The model under review builds one solid part; all positions refer to its coordinate system, in mm. Give positions to 0.01 mm unless a question says otherwise; leave off trailing zeros. Order: outer loops, then holes, each group sorted by start corner. A loop starts at its lowest first (then second) coordinate and runs counter-clockwise, first axis right, second up.
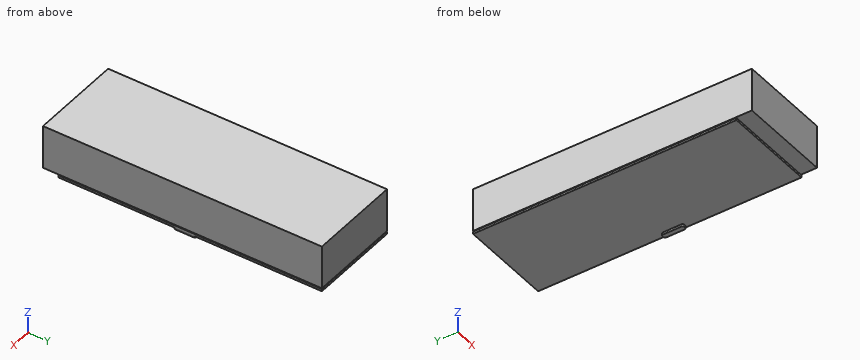
Autodesk Inventor part; units mm, degrees
ref_plane "YZ Plane" through (0, 0, 0) normal (1, 0, 0) x (0, 1, 0)
ref_plane "XZ Plane" through (0, 0, 0) normal (0, 1, 0) x (-1, 0, 0)
ref_plane "XY Plane" through (0, 0, 0) normal (0, 0, 1) x (1, 0, 0)
sketch "Skizze1" plane through (0, 0, 0) normal (0, 1, 0) x (-1, 0, 0)
  line L0 (0, 0) -> (600, 0)
  line L1 (600, 0) -> (600, -280)
  line L2 (600, -280) -> (0, -280)
  line L3 (0, -280) -> (0, 0)
  dimension "d0" = 600
  dimension "d1" = 280
extrude "Extrusion1" add sketch "Skizze1" along normal blind 1800
sketch "Skizze2" plane through (0, 0, -280) normal (0, 0, -1) x (-1, 0, 0)
  line L0 (10, 1790) -> (590, 1790)
  line L1 (590, 1790) -> (590, 110)
  line L2 (590, 110) -> (10, 110)
  line L3 (10, 110) -> (10, 1790)
  line L4 (0, 0) -> (0, 1800)
  line L5 (600, 0) -> (600, 1800)
  line L6 (0, 1800) -> (600, 1800)
  line L7 (0, 0) -> (600, 0)
  dimension "d4" = 10
  dimension "d5" = 10
  dimension "d6" = 10
  dimension "d7" = 110
extrude "Extrusion2" add sketch "Skizze2" along normal blind 5 contours L0 L1 L2 L3
sketch "Skizze3" plane through (0, 0, -285) normal (0, 0, -1) x (-1, 0, 0)
  line L0 (0, 0) -> (0, 1800)
  line L1 (600, 0) -> (600, 1800)
  line L2 (0, 1800) -> (600, 1800)
  line L3 (600, 1800) -> (600, 100)
  line L4 (600, 100) -> (0, 100)
  line L5 (0, 100) -> (0, 1800)
  line L6 (10, 110) -> (590, 110)
  point P0 (0, 100)
  dimension "d10" = 10
extrude "Extrusion3" add sketch "Skizze3" along normal blind 15
sketch "Skizze4" plane through (0, 0, -300) normal (0, 0, -1) x (-1, 0, 0)
  line L0 (15, 980) -> (25, 980)
  line L1 (35, 970) -> (35, 850)
  line L2 (25, 840) -> (15, 840)
  line L3 (5, 850) -> (5, 970)
  line L4 (0, 0) -> (600, 0)
  line L5 (0, 1800) -> (0, 100)
  arc A0 (5, 850) -> (15, 840) centre (15, 850) ccw
  arc A1 (25, 840) -> (35, 850) centre (25, 850) ccw
  arc A2 (35, 970) -> (25, 980) centre (25, 970) ccw
  arc A3 (15, 980) -> (5, 970) centre (15, 970) ccw
  dimension "d13" = 840
  dimension "d14" = 140
  dimension "d15" = 30
  dimension "d16" = 5
  dimension "d17" = 10
extrude "Extrusion4" add sketch "Skizze4" along normal blind 15
equation "\"d5\" = d4"
equation "\"d6\" = d5"
properties part number "Schaltschrank1"
Item 1: Clearance check with flat-ended pins moving along their axes: pin 1 Ø11 at (x, z) = (-21.5, -310) entering from -Y; pin 2 Ø8 at (x, z) = (-20.5, -305.5) entering from +Y; pin 3 Ø7.5 at (x, z) = (-183, -296) entering from -Y. State where each tip first meets the part, or that it passes through.
Values found:
pin 1: stops at y = 840
pin 2: stops at y = 980
pin 3: stops at y = 100
Item 2: Take a section at A-A (x = -173.5). Give the boundary of the cut face in (y, z).
Values found:
outline: (0, -280) - (110, -280) - (110, -285) - (100, -285) - (100, -300) - (1800, -300) - (1800, -285) - (1790, -285) - (1790, -280) - (1800, -280) - (1800, 0) - (0, 0) - close
Item 3: For line 1 (Z direction, x = -292, y = 521); line 2 (Y direction, x = -182.5, z = -282.5); line 3 (X direction, y = 635, z = -284), list the stretches that pass through material, from the lowest coordinate up.
Values found:
line 1: z = -300 to 0
line 2: y = 110 to 1790
line 3: x = -590 to -10
Item 4: Take a section at B-B (y = 664). Give the boundary of the cut face in (x, z), and give its area (3 significant figures).
Values found:
outline: (-600, -300) - (0, -300) - (0, -285) - (-10, -285) - (-10, -280) - (0, -280) - (0, 0) - (-600, 0) - (-600, -280) - (-590, -280) - (-590, -285) - (-600, -285) - close
area: 180,000 mm2
